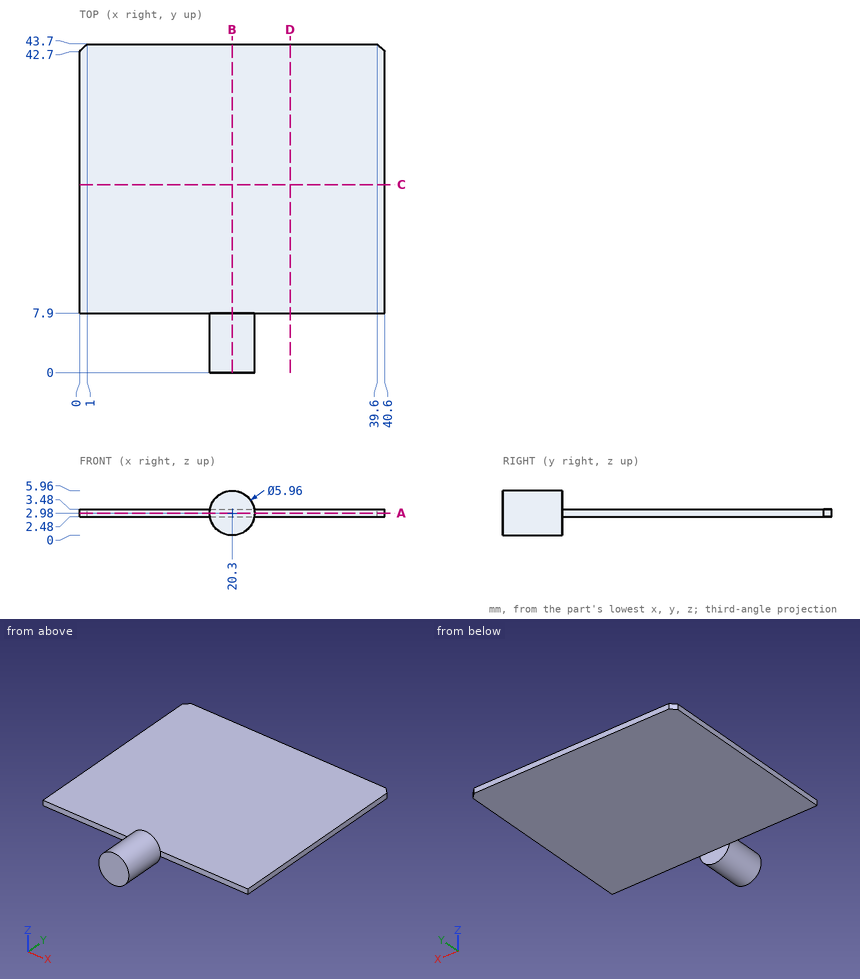
Check sheet for the drawn part. Datum: minimum x, y, z corner. Units: mm. Coordinates: 2 decimals unless noted, no trailing zeros. Order: outer loops, then holes, each group sorted by start corner. A loop starts at its lowest first (then second) coordinate and runs counter-clockwise, first axis right, second up. Notation, with made-up numbers: (40.5, 33) -> (49.5, 33) arc R21 ccw to (49.5, 45) -> close; hole circle Ø2 at (39.25, -4.75). An arc over 180 degrees is marked (long way). Use a Markdown table: item, result. Add a question column.
1. Go/stop test with flat-tipped pins: pin 1 Ø0.8 at (x, z) = (11.5, 3) entering from -Y; pin 2 Ø1.2 at (x, z) = (21.5, 0.5) entering from +Y; pin 3 Ø8 at (x, y) = (22, 20) entering from +Z. Record where each tip stops, or that it passes through.
2. Cross-section at D-D (x = 28). Enter the section's corners in (y, z), and give its area (3 significant figures).
3. Cross-section at A-A (z = 2.98). Enter the section's corners in (x, y), and give its area (3 significant figures).
4. Cross-section at C-C (y = 25). Enter the section's corners in (x, z), and give its area (3 significant figures).
5. Material ranges on L1, parallel to Z at x = 6, y = 30; L2, parallel to Y at x = 37, z = 3.25; L3, parallel to Y at x = 20, z = 1.7, recorded low to high.
6. Cross-section at B-B (x = 20.3). Enter the section's corners in (y, z).
Filled sheet:
| question | item | result |
|---|---|---|
| 1 | pin 1 | y = 7.9 |
| 1 | pin 2 | y = 7.9 |
| 1 | pin 3 | z = 3.48 |
| 2 | outline | (7.9, 2.48) -> (43.7, 2.48) -> (43.7, 3.48) -> (7.9, 3.48) -> close |
| 2 | area | 35.8 mm2 |
| 3 | outline | (0, 7.9) -> (17.32, 7.9) -> (17.32, 0) -> (23.28, 0) -> (23.28, 7.9) -> (40.6, 7.9) -> (40.6, 42.7) -> (39.6, 43.7) -> (1, 43.7) -> (0, 42.7) -> close |
| 3 | area | 1,500 mm2 |
| 4 | outline | (0, 2.48) -> (40.6, 2.48) -> (40.6, 3.48) -> (0, 3.48) -> close |
| 4 | area | 40.6 mm2 |
| 5 | L1 | 2.48 to 3.48 |
| 5 | L2 | 7.9 to 43.7 |
| 5 | L3 | 0 to 7.9 |
| 6 | outline | (0, 0) -> (7.9, 0) -> (7.9, 2.48) -> (43.7, 2.48) -> (43.7, 3.48) -> (7.9, 3.48) -> (7.9, 5.96) -> (0, 5.96) -> close |
